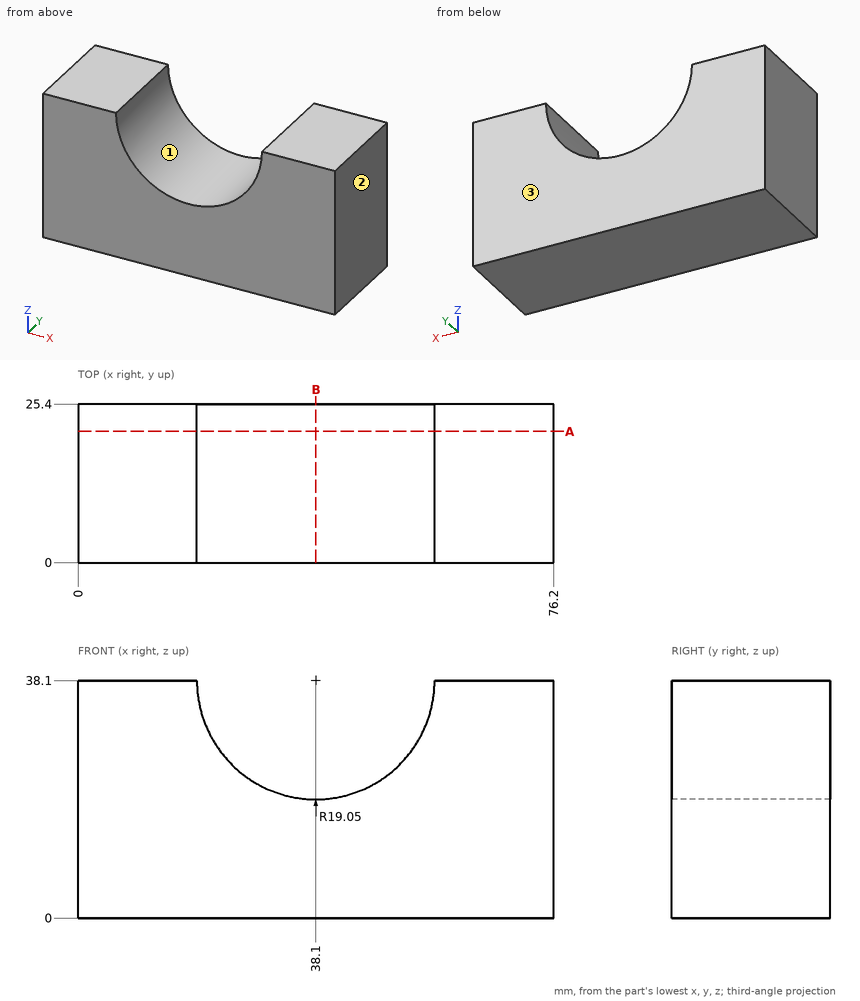
Drawing for the job (mm, zero at the part's lowest x, y, z). Give positions to 0.01 mm unless a question says otherwise; leave off trailing zeros. Loops run counter-clockwise (first coordinate to the right, second up) from the corner with the lowest first, then second, coordinate; pieces in that order, holes last.
Item 1: Drill centre lines: line 1 along X through (y, z) = (1.5, 22); line 2 along X through (y, z) = (8, 25); line 3 along Z through (x, y) = (31.5, 2.5). Where is each one in solid material? Low to high.
Check values:
line 1: x = 0 to 27.92, 48.28 to 76.2
line 2: x = 0 to 24.27, 51.93 to 76.2
line 3: z = 0 to 20.23
Item 2: Mould opens along X. For the marked faces 1, 2 and 3 say: +X half, -X half, draft (parallel to the pull), parting line (faces both ways), or undercut.
Check values:
face 1: undercut
face 2: +X half
face 3: draft
Item 3: Drop flat-ended pins along their axis: P1, Ø3, axis at x = 35, y = 14, coming from the -Z side; P2, Ø8, axis at x = 30, y = 6.5, coming from the +Z side; P3, Ø4, axis at x = 26, y = 8.5, coming from the +Z side; P4, Ø12, axis at x = 27.5, y = 12.5, coming from the +Z side. Give the stop position or say it passes through.
Check values:
P1: stops at z = 0
P2: stops at z = 23.39
P3: stops at z = 25.29
P4: stops at z = 28.75
Item 4: Slice it at B-B (x = 38.1). Write the cut outline in (y, z).
Check values:
outline: (0, 0) - (25.4, 0) - (25.4, 19.05) - (0, 19.05) - close
Item 5: Slice it at A-A (y = 21). Write the cut outline in (x, z), plus the area to 3 significant figures.
Check values:
outline: (0, 0) - (76.2, 0) - (76.2, 38.1) - (57.15, 38.1) arc R19.05 cw to (19.05, 38.1) - (0, 38.1) - close
area: 2,330 mm2
